```python
from build123d import *

# Parameters (mm, degrees)
BOSS_EXTRUDE1_DEPTH         = 12.7
CUT_EXTRUDE1_DEPTH          = 13.7
SKETCH3_W                   = 28.575
SKETCH3_H                   = 12.7
F_8_CLEARANCE_HOLE1_D       = 4.5
F_8_CLEARANCE_HOLE1_DEPTH   = 12.7
F_1_4_CLEARANCE_HOLE1_D     = 6.6
F_1_4_CLEARANCE_HOLE1_DEPTH = 12.7
F_12_CLEARANCE_HOLE1_D      = 6
F_12_CLEARANCE_HOLE1_DEPTH  = 12.7
HOLE1_D                     = 6.4
HOLE1_DEPTH                 = 24.77643101
HOLE1_CBORE_D               = 11.2
HOLE1_CBORE_DEPTH           = 11.77643101
F_10_CLEARANCE_HOLE1_D      = 5
F_10_CLEARANCE_HOLE1_DEPTH  = 36.4125
CHAMFER1_SIZE               = 3
SKETCH14_R                  = 3
SKETCH14_R_2                = 1.651
BOSS_EXTRUDE2_DEPTH         = 12.7


with BuildPart() as part:
    # Sketch1 → Boss-Extrude1 (new body)
    with BuildSketch(Plane(origin=(0, 0, 0), x_dir=(-1, 0, 0), z_dir=(0, 0, -1))):
        with BuildLine():
            Line((224.169455465, 127.72254562), (151.435240745, 147.211619716))
            ThreePointArc((151.435240745, 147.211619716), (105.257753851, 121.607458019), (129.246532787, 74.570537656))
            Line((129.246532787, 74.570537656), (211.469455465, 46.304993078))
            Line((211.469455465, 46.304993078), (224.169455465, 46.304993078))
            Line((224.169455465, 46.304993078), (224.169455465, 127.72254562))
        make_face()
    extrude(amount=-BOSS_EXTRUDE1_DEPTH)

    # Sketch2 → Cut-Extrude1 (cut, through all)
    with BuildSketch(Plane.XY.offset(12.7)):
        with BuildLine():
            Line((-103.633291463, 112.093938317), (-113.179018515, 112.093938317))
            ThreePointArc((-113.179018515, 112.093938317), (-113.134717032, 110.506438317), (-113.179018515, 108.918938317))
            Line((-113.179018515, 108.918938317), (-103.633291463, 108.918938317))
            ThreePointArc((-103.633291463, 108.918938317), (-103.600117032, 110.506438317), (-103.633291463, 112.093938317))
        make_face()
    extrude(amount=-CUT_EXTRUDE1_DEPTH, mode=Mode.SUBTRACT)

    # Sketch3 → Cut-Revolve1 (revolve, cut)
    with BuildSketch(Plane(origin=(0, 110.506438317, 0), x_dir=(1, 0, 0), z_dir=(0, 1, 0))):
        with Locations((-127.312617032, -6.35)):
            Rectangle(SKETCH3_W, SKETCH3_H)
    revolve(axis=Axis((-141.600117032, 110.506438317, 0), (0, 0, 1)), mode=Mode.SUBTRACT)

    # #8 Clearance Hole1
    with Locations(Plane.XY.offset(12.7)):
        with Locations((-117.978117032, 86.884438317), (-165.222117032, 86.884438317), (-165.222117032, 134.128438317), (-117.978117032, 134.128438317)):
            Hole(F_8_CLEARANCE_HOLE1_D / 2, depth=F_8_CLEARANCE_HOLE1_DEPTH)

    # 1/4 Clearance Hole1
    with Locations(Plane(origin=(0, 0, 0), x_dir=(-1, 0, 0), z_dir=(0, 0, -1))):
        with Locations((217.819455465, 53.304993078), (217.819455465, 76.304993078), (217.819455465, 99.304993078)):
            Hole(F_1_4_CLEARANCE_HOLE1_D / 2, depth=F_1_4_CLEARANCE_HOLE1_DEPTH)

    # #12 Clearance Hole1
    with Locations(Plane.XY.offset(12.7)):
        with Locations((-192.169455465, 89.72254562)):
            Hole(F_12_CLEARANCE_HOLE1_D / 2, depth=F_12_CLEARANCE_HOLE1_DEPTH)

    # Hole1
    with Locations(Plane(origin=(0, 84.142507307, 0), x_dir=(-1, 0, 0), z_dir=(0, -1, 0))):
        with Locations((108.633291463, -6.35)):
            CounterBoreHole(HOLE1_D / 2, HOLE1_CBORE_D / 2, HOLE1_CBORE_DEPTH, depth=HOLE1_DEPTH)

    # #10 Clearance Hole1
    with Locations(Plane(origin=(0, 112.093938317, 0), x_dir=(-1, 0, 0), z_dir=(0, -1, 0))):
        with Locations((108.633291463, -6.35)):
            Hole(F_10_CLEARANCE_HOLE1_D / 2, depth=F_10_CLEARANCE_HOLE1_DEPTH)

    # Chamfer1
    chamfer1_edges = [part.edges().sort_by_distance(p)[0] for p in [
        (-221.119455465, 99.304993078, 0),
        (-221.119455465, 76.304993078, 0),
        (-221.119455465, 53.304993078, 0),
    ]]
    chamfer(chamfer1_edges, length=CHAMFER1_SIZE)

    # Sketch14 → Boss-Extrude2 (add)
    with BuildSketch(Plane(origin=(0, 0, 0), x_dir=(-1, 0, 0), z_dir=(0, 0, -1))):
        with Locations((192.169455465, 89.72254562)):
            Circle(SKETCH14_R)
        with Locations((192.169455465, 89.72254562)):
            Circle(SKETCH14_R_2, mode=Mode.SUBTRACT)
    extrude(amount=-BOSS_EXTRUDE2_DEPTH)


solid = part.part
```
Verification items for the finished model (mm, model axes). Give positions to 0.01 mm unless a question says otherwise; leave off trailing zeros. Order: outer loops, then holes, each group sorted by start corner. A loop starts at its lowest first (then second) coordinate and runs counter-clockwise, first axis right, second up. Notation, with made-up numbers: (88.25, 81) - (136.25, 81) arc R13 ccw to (136.25, 102) - close; hole circle Ø9 at (28.25, 16). An arc over 180 degrees is marked (long way). Answer as CSV lines item,"result". Start each with the question number.
Item 1: Material ranges on L1, parallel to X at y = 101.5, z = 3.75; L2, parallel to Y at x = -126, z = 5; L3, parallel to X at y = 98, z = 7.5, recorded low to high.
Item 2: Section check B-B, the plane x = -157. Record the boundary of the cut face in (y, z).
Item 3: Section check A-A, the plane z = 6.35. State how many separate pieces and enclosed holes the cut face has, plus the area to 3 significant figures.
Item 4: Mould release check, pull along X, two halves, no side actions. Record for faces 1 (the face through (-216.05, 79.09, 7.92)), 2 (the face through (-169.782, 60.636, 6.261)), 3 (the face through (-176, 98, 0)): released by +X, released by -X, zero draft, split by the parting line, or undercut.
Item 5: Section check C-C, the plane x = -141. Record the boundary of the cut face in (y, z).
Item 6: Gauge pin test, flat ends, axial feed: pin 1 (3 mm diameter, centred on x = -166, z = 2.5, fed in from -Y); pin 2 (6 mm diameter, centred on y = 138, z = 10.5, fed in from +X); pin 3 (2.5 mm diameter, centred on x = -110.5, z = 6.5, fed in from -Y). Record the tip position at first contact, or that the pin passes through.
Filled in:
1,L1,"-224.17 to -220.28, -215.36 to -168.72, -114.48 to -110.5, -106.77 to -104.68"
1,L2,"75.86 to 86.57, 134.45 to 145.16"
1,L3,"-224.17 to -220.85, -214.79 to -167.29, -115.91 to -111.62"
2,outline,"(65.03, 0) - (86.44, 0) - (86.44, 12.7) - (65.03, 12.7) - close; (134.58, 0) - (145.72, 0) - (145.72, 12.7) - (134.58, 12.7) - close"
3,separate pieces,"3"
3,enclosed holes,"8"
3,area,"6,080 mm^2"
4,face 1,"undercut"
4,face 2,"released by +X"
4,face 3,"zero draft"
5,outline,"(70.53, 0) - (81.94, 0) - (81.94, 12.7) - (70.53, 12.7) - close; (139.08, 0) - (148.5, 0) - (148.5, 12.7) - (139.08, 12.7) - close"
6,pin 1,"y = 61.42"
6,pin 2,"x = -112.55"
6,pin 3,"y = 112.09"
